```python
from build123d import *

# Parameters (mm, degrees)
SKETCH1_R           = 14
BOSS_EXTRUDE1_DEPTH = 9
SKETCH2_OUTSIDE_W   = 38.122
SKETCH2_OUTSIDE_H   = 38.122
SKETCH2_OUTSIDE_W_2 = 22
SKETCH2_OUTSIDE_H_2 = 28
CUT_EXTRUDE1_DEPTH  = 22.748563171
SKETCH3_R           = 2.5
CUT_EXTRUDE2_DEPTH  = 20.949937343
CHAMFER1_SIZE       = 2
BOSS_EXTRUDE2_START = 3
SKETCH4_W           = 11
SKETCH4_H           = 12.339745962
BOSS_EXTRUDE2_DEPTH = 3.5
SKETCH5_R           = 1.625
CUT_EXTRUDE3_DEPTH  = 26.357444666
CUT_EXTRUDE4_START  = 3
CUT_EXTRUDE4_DEPTH  = 3.5
CIRPATTERN1_COUNT   = 2
FILLET1_R           = 2
SKETCH7_R           = 1.5
CUT_EXTRUDE5_DEPTH  = 2.5


# Read off the part's stored shape, not the designer's step: Cut-Extrude4
with BuildPart() as part:
    # Sketch1 → Boss-Extrude1 (new body)
    with BuildSketch(Plane.XY):
        Circle(SKETCH1_R)
    extrude(amount=BOSS_EXTRUDE1_DEPTH)

    # Sketch2 outside → Cut-Extrude1 (cut, through all)
    with BuildSketch(Plane.XY):
        Rectangle(SKETCH2_OUTSIDE_W, SKETCH2_OUTSIDE_H)
        Rectangle(SKETCH2_OUTSIDE_W_2, SKETCH2_OUTSIDE_H_2, mode=Mode.SUBTRACT)
    extrude(amount=CUT_EXTRUDE1_DEPTH, mode=Mode.SUBTRACT)

    # Sketch3 → Cut-Extrude2 (cut, through all)
    with BuildSketch(Plane.XY.offset(9)):
        Circle(SKETCH3_R)
    extrude(amount=-CUT_EXTRUDE2_DEPTH, mode=Mode.SUBTRACT)

    # Chamfer1
    chamfer1_edges = [part.edges().sort_by_distance(p)[0] for p in [
        (-2.5, 0, 9),
    ]]
    chamfer(chamfer1_edges, length=CHAMFER1_SIZE)

    # Sketch4 → Boss-Extrude2 (add)
    with BuildSketch(Plane.XY.offset(BOSS_EXTRUDE2_START)):
        with Locations((5.5, 14.830127019)):
            Rectangle(SKETCH4_W, SKETCH4_H)
    boss_extrude2 = extrude(amount=BOSS_EXTRUDE2_DEPTH)

    # Sketch5 → Cut-Extrude3 (cut, through all)
    with BuildSketch(Plane.XY):
        with Locations((6, 16.5)):
            Circle(SKETCH5_R)
    cut_extrude3 = extrude(amount=CUT_EXTRUDE3_DEPTH, mode=Mode.SUBTRACT)

    # Cut-Extrude4 outline → Cut-Extrude4 (cut)
    with BuildSketch(Plane.XY.offset(CUT_EXTRUDE4_START)):
        with BuildLine():
            Line((11, 21), (0, 21))
            ThreePointArc((0, 21), (5.715793024, 20.20716977), (11, 17.88854382))
            Line((11, 17.88854382), (11, 21))
        make_face()
    cut_extrude4 = extrude(amount=CUT_EXTRUDE4_DEPTH, mode=Mode.SUBTRACT)

    # CirPattern1: Boss-Extrude2, Cut-Extrude3, Cut-Extrude4 ×2 about axis
    cirpattern1_axis = Axis((0, 0, 0), (0, 0, 1))
    add([boss_extrude2.rotate(cirpattern1_axis, i * 360 / CIRPATTERN1_COUNT) for i in range(1, CIRPATTERN1_COUNT)])
    add([cut_extrude3.rotate(cirpattern1_axis, i * 360 / CIRPATTERN1_COUNT) for i in range(1, CIRPATTERN1_COUNT)], mode=Mode.SUBTRACT)
    add([cut_extrude4.rotate(cirpattern1_axis, i * 360 / CIRPATTERN1_COUNT) for i in range(1, CIRPATTERN1_COUNT)], mode=Mode.SUBTRACT)

    # Fillet1
    fillet1_edges = [part.edges().sort_by_distance(p)[0] for p in [
        (-11, -17.88854382, 4.75),
        (0, 21, 4.75),
        (11, 17.88854382, 4.75),
        (0, -21, 4.75),
    ]]
    fillet(fillet1_edges, radius=FILLET1_R)

    # Sketch7 → Cut-Extrude5 (cut)
    with BuildSketch(Plane.XY.offset(9)):
        with Locations((3, -13.674794331)):
            Circle(SKETCH7_R)
    extrude(amount=-CUT_EXTRUDE5_DEPTH, mode=Mode.SUBTRACT)


solid = part.part
```
Model file for the job. Use its own axes, mm. A direction names the side the tool comes from. Coordinates: 2 decimals unless noted, no trailing zeros. Write each loop counter-clockwise with the first axis right and the second up, starting at its lowest first coordinate (ties: lowest second). Pieces come first, ordered by that corner, then holes. Notation, with made-up numbers: (85, 8) - (144, 8) arc R27 ccw to (144, 46) - close; hole circle Ø11 at (6, 15). An arc over 180 degrees is marked (long way). One line per item, written item: value. Start each with the question number.
1. Slice it at B-B (x = 6). Write the cut outline in (y, z) (3 decimals), plus the area to 3 significant figures.
2. Probe line 1 (Y direction, x = 5, z = 4.25); line 2 (X direction, y = -11, z = 3.25); line 3 (Y direction, x = 6, z = 4.55) (3 decimals). List the from-to ranges inside material, lowest first. Write a range as from..to.
3. Mould opens along Y. For faces 1 (the flat face through (0, 16, 5)), 2 (the cylindrical face through (-0.645, -20.365, 4.774)), 3 (the cylindrical face through (0.68, 20.397, 4.774)), 4 (the cylindrical face through (-0.54, -2.44, 3.55)) say: released by +Y, released by -Y, zero draft, split by the parting line, or undercut.
4. Tool access for faces 5 (the flat face through (-5, -15, 3)), 6 (the flat face through (-3, 0, 0)), 7 (the flat face through (-5, -15, 6.5)), 8 (the flat face through (0, -16, 5)), 9 (the flat face through (-5, 0, 9)): list every direction of +Z, -Z, +X, -X, +Y, -Y with a clear straight run to the whole face (end or side of a thin tool).
5. Slice it at A-A (y = 0). Write the cut outline in (x, z), plus the area to 3 significant figures.
6. Slice it at D-D (y = 12). Write the cut outline in (x, z), plus the area to 3 significant figures.
7. Flat gauge pins, fed straight in: pin 1 (1 mm diameter, centred on x = -6, y = 14, fed in from +Z); pin 2 (4 mm diameter, centred on x = -6, y = -16.5, fed in from -Z); pin 3 (0.9 mm diameter, centred on x = 2.5, y = -13.5, fed in from +Z); pin 4 (5 mm diameter, centred on x = -6, y = 14.5, fed in from -Z). Where does each tip first touch, or does it go through?
8. Slice it at C-C (z = 0.75). Write the cut outline in (x, y).
Answers below:
1. outline: (-12.649, 0) - (12.649, 0) - (12.649, 3) - (14.875, 3) - (14.875, 6.5) - (12.649, 6.5) - (12.649, 9) - (-12.649, 9) - close; (18.125, 3) - (20.125, 3) - (20.125, 6.5) - (18.125, 6.5) - close
1. area: 242 mm^2
2. line 1: y = -13.08..15.22, 17.78..20.4
2. line 2: x = -11..8.66
2. line 3: y = -12.649..14.875, 18.125..20.125
3. face 1: zero draft
3. face 2: released by -Y
3. face 3: released by +Y
3. face 4: undercut
4. face 5: -Z, -X, -Y
4. face 6: -Z, +X, -X, +Y, -Y
4. face 7: +Z, -X, -Y
4. face 8: +Z, -Z, +X, -Y
4. face 9: +Z, +X, -X, +Y, -Y
5. outline: (-11, 0) - (-2.5, 0) - (-2.5, 7) - (-4.5, 9) - (-11, 9) - close; (2.5, 0) - (11, 0) - (11, 9) - (4.5, 9) - (2.5, 7) - close
5. area: 149 mm^2
6. outline: (-7.21, 0) - (7.21, 0) - (7.21, 3) - (11, 3) - (11, 6.5) - (7.21, 6.5) - (7.21, 9) - (-7.21, 9) - close
6. area: 143 mm^2
7. pin 1: passes through
7. pin 2: stops at z = 3
7. pin 3: stops at z = 6.5
7. pin 4: stops at z = 0
8. outline: (-11, -8.66) arc R14 ccw to (11, -8.66) - (11, 8.66) arc R14 ccw to (-11, 8.66) - close; hole circle Ø5 at (0, 0)
